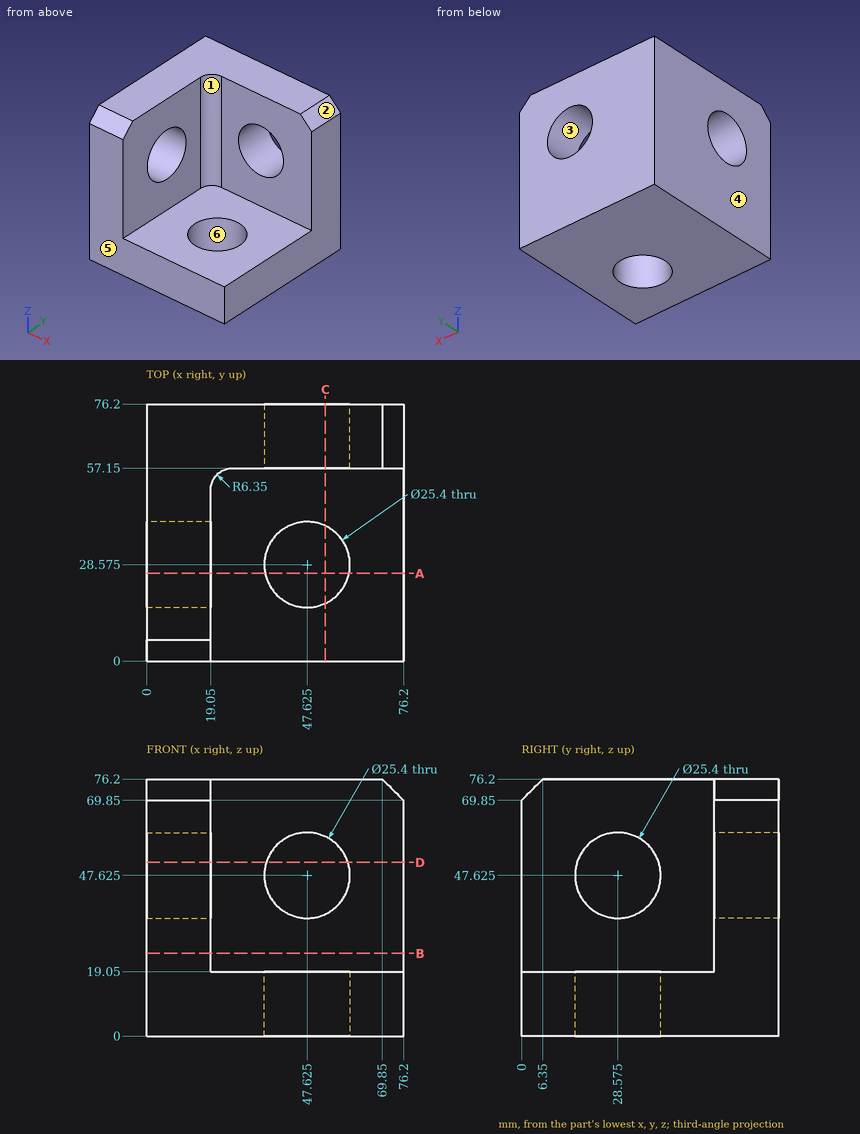
Print and shaded views of the part. All mm, measured from the part's lowest x, y and z. A direction names the side the tool comes from. Coordinates: 2 decimals unless noted, no trailing zeros. Loops run counter-clockwise (first coordinate to the right, second up) from the corner with the lowest first, then second, coordinate; pieces in that order, holes last. Notation, with made-up numbers: (83, 4) - (136, 4) arc R37 cw to (136, 40) - close; hole circle Ø11 at (49.5, -10.75). An arc over 180 degrees is marked (long way). Write item = value, one per line. Start each with the question number.
Item 1: Cut at B-B, the plane z = 24.5. Give the cut face in (x, y), and give its area (3 significant figures).
Item 2: Mould opens along X. For the marked faces 3, 4, 5 and 6 say: released by +X, released by -X, zero draft, split by the parting line, or undercut.
Item 3: Cut at A-A, the plane y = 26. Give the cut face in (x, z), and give its area (3 significant figures).
Item 4: Flat gauge pins, fed straight in: pin 1 Ø6 at (x, y) = (37, 18) entering from +Z; pin 2 Ø12 at (y, z) = (20, 36) entering from -X; pin 3 Ø4 at (y, z) = (33.5, 62.5) entering from +X; pin 4 Ø15 at (x, y) = (47.625, 28.575) entering from -Z. Where does each tip first touch, or does it go through?
Item 5: Wall check: L1, parallel to Z at x = 48, y = 60.5; L2, parallel to Z at x = 42.5, y = 50. Give the ranges that are in metal, low to high. Write a range as from..to.
Item 6: Cut at D-D, the plane z = 51.5. Give the cut face in (x, y), and give its area (3 significant figures).
Item 7: Cut at C-C, the plane x = 53. Give the cut face in (y, z), and give its area (3 significant figures).
Item 8: 3-axis set-ups, long thin cutter, end or side, ignore diameter. For the marked faces 1 and 2: which of +Z, -Z, +X, -X, +Y, -Y reach the whole face in a straight line?
The answers:
q1.outline = (0, 0) - (19.05, 0) - (19.05, 50.8) arc R6.35 cw to (25.4, 57.15) - (76.2, 57.15) - (76.2, 76.2) - (0, 76.2) - close
q1.area = 2,550 mm2
q2.face_3 = undercut
q2.face_4 = released by -X
q2.face_5 = zero draft
q2.face_6 = undercut
q3.outline = (0, 0) - (35.19, 0) - (35.19, 19.05) - (19.05, 19.05) - (19.05, 35.19) - (0, 35.19) - close; (0, 60.06) - (19.05, 60.06) - (19.05, 76.2) - (0, 76.2) - close; (60.06, 0) - (76.2, 0) - (76.2, 19.05) - (60.06, 19.05) - close
q3.area = 1,590 mm2
q4.pin_1 = 19.05
q4.pin_2 = 0
q4.pin_3 = 19.05
q4.pin_4 = through
q5.L1 = 0..34.93, 60.32..76.2
q5.L2 = 0..19.05
q6.outline = (0, 0) - (19.05, 0) - (19.05, 16.48) - (0, 16.48) - close; (0, 40.67) - (19.05, 40.67) - (19.05, 50.8) arc R6.35 cw to (25.4, 57.15) - (35.53, 57.15) - (35.53, 76.2) - (0, 76.2) - close; (59.72, 57.15) - (76.2, 57.15) - (76.2, 76.2) - (59.72, 76.2) - close
q6.area = 1,630 mm2
q7.outline = (0, 0) - (17.07, 0) - (17.07, 19.05) - (0, 19.05) - close; (40.08, 0) - (76.2, 0) - (76.2, 36.12) - (57.15, 36.12) - (57.15, 19.05) - (40.08, 19.05) - close; (57.15, 59.13) - (76.2, 59.13) - (76.2, 76.2) - (57.15, 76.2) - close
q7.area = 1,660 mm2
q8.face_1 = +Z, +X, -Y
q8.face_2 = +Z, +X, +Y, -Y
